Verification items for this drawing (mm, ordinates from the low corner). A direction names the side the tool comes from. Coordinates: 2 decimals unless noted, no trailing zeros. Write each loop counter-clockwise with the first axis right and the second up, starting at its lowest first coordinate (ties: lowest second). Pieces come first, ordered by that corner, then holes.
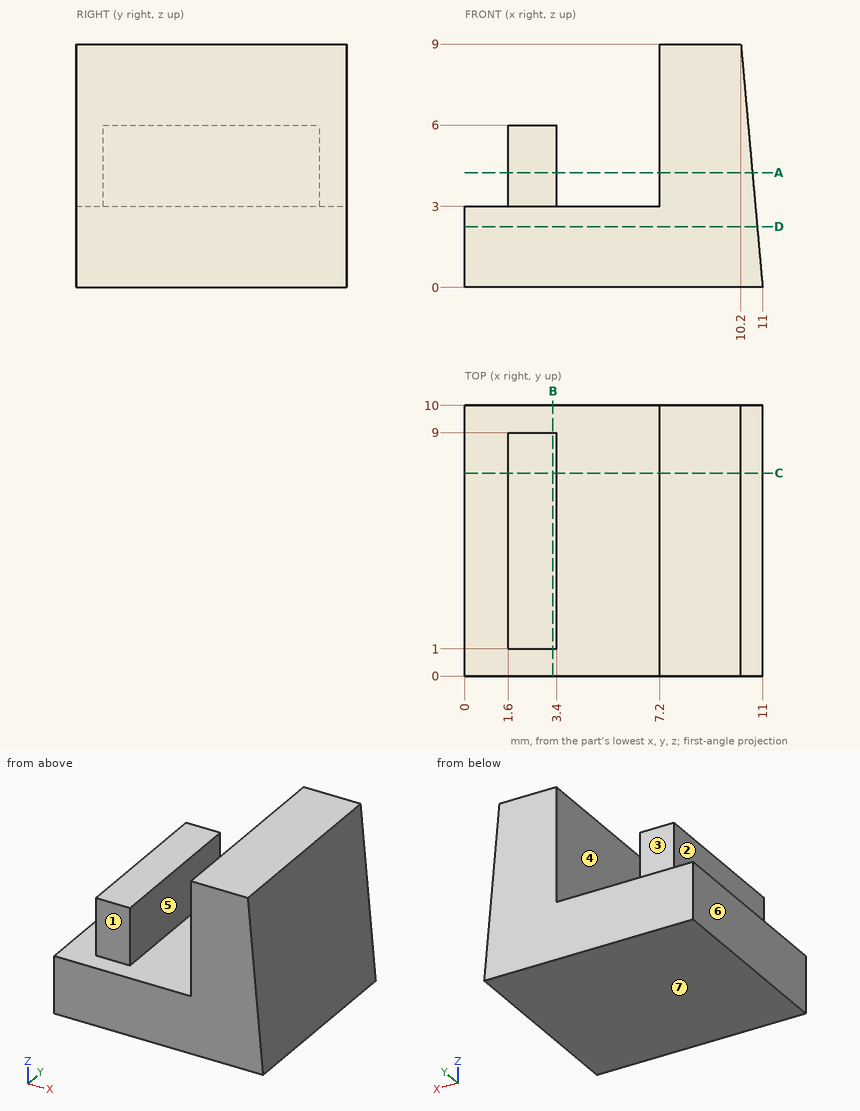
1. Access from +Z, -Z, +X, -X, +Y, -Y to the whole of each face (thin tool, end or side, straight path). Record for the marked faces 1, 2 and 3.
Computed values:
face 1: +Z, -X, -Y
face 2: +Z, -X, +Y, -Y
face 3: +Z, -X, +Y
2. Sectioned sample at C-C, the plane y = 7.5. Record the boundary of the cut face in (x, z), and give its area (3 significant figures).
Computed values:
outline: (0, 0) - (11, 0) - (10.2, 9) - (7.2, 9) - (7.2, 3) - (3.4, 3) - (3.4, 6) - (1.6, 6) - (1.6, 3) - (0, 3) - close
area: 57.6 mm2
3. Sectioned sample at A-A, the plane z = 4.25. Record the boundary of the cut face in (x, y).
Computed values:
outline: (1.6, 1) - (3.4, 1) - (3.4, 9) - (1.6, 9) - close; (7.2, 0) - (10.62, 0) - (10.62, 10) - (7.2, 10) - close
4. Sectioned sample at D-D, the plane z = 2.25. Record the boundary of the cut face in (x, y), and give its area (3 significant figures).
Computed values:
outline: (0, 0) - (10.8, 0) - (10.8, 10) - (0, 10) - close
area: 108 mm2
5. Draft check along X on the marked faces 4, 5, 6 and 7. Enter one of: released by +X, released by -X, zero draft, split by the parting line, or undercut.
Computed values:
face 4: undercut
face 5: undercut
face 6: released by -X
face 7: zero draft
6. Sectioned sample at B-B, the plane x = 3.25. Record the boundary of the cut face in (y, z).
Computed values:
outline: (0, 0) - (10, 0) - (10, 3) - (9, 3) - (9, 6) - (1, 6) - (1, 3) - (0, 3) - close
7. Thickness scan on line 1 along Z through (x, y) = (2.25, 9.75); line 2 along X through (y, z) = (6, 4); line 3 along Z through (x, y) = (2.5, 3). Record the ranges inside material, lowest first.
Computed values:
line 1: z = 0 to 3
line 2: x = 1.6 to 3.4, 7.2 to 10.64
line 3: z = 0 to 6
8. Gauge pin test, flat ends, axial feed: pin 1 Ø0.9 at (x, z) = (2, 4.5) entering from +Y; pin 2 Ø6 at (x, y) = (6, 1.5) entering from -Z; pin 3 Ø0.9 at (x, y) = (3, 3) entering from +Z; pin 4 Ø1.5 at (y, z) = (6.5, 4.5) entering from -X. Record the tip position at first contact, or that the pin passes through.
Computed values:
pin 1: stops at y = 9
pin 2: stops at z = 0
pin 3: stops at z = 6
pin 4: stops at x = 1.6
